Build history of the part. All positions in model axes, mm. A direction names the side the tool comes from. Give positions to 0.01 mm unless a question says otherwise; leave off trailing zeros. Loops run counter-clockwise (first coordinate to the right, second up) from the corner with the lowest first, then second, coordinate; pieces in that order, holes last. Notation, with made-up numbers: (-24.75, 6) -> (34.25, 6) arc R13 ccw to (34.25, 21) -> close; hole circle Ø3 at (44, 37.25). An arc over 180 degrees is marked (long way). Answer as a JSON object with one key per item and string values. Group by question number.
from build123d import *

# Parameters (mm, degrees)
F0_R     = 2.5
F1_DEPTH = 10
F2_DEPTH = 10
F3_R     = 1


with BuildPart() as f1:
    # F0 (on Top) → F1 (new body)
    with BuildSketch(Plane.XY):
        Polygon((-4.778127, 51.351744), (-24.778127, 51.351744), (-24.778127, -18.648256), (40.221873, -18.648256), (40.221873, 51.351744), (20.221873, 51.351744), (20.221873, 1.351744), (-4.778127, 1.351744), align=None)
        with Locations((-14.778127, 18.851744)):
            Circle(F0_R, mode=Mode.SUBTRACT)
        with Locations((30.221873, 18.851744)):
            Circle(F0_R, mode=Mode.SUBTRACT)
    extrude(amount=F1_DEPTH)

    # F0 (on Top) → F2 (join)
    with BuildSketch(Plane.XY):
        Polygon((-4.778127, 51.351744), (-24.778127, 51.351744), (-24.778127, -18.648256), (40.221873, -18.648256), (40.221873, 51.351744), (20.221873, 51.351744), (20.221873, 1.351744), (-4.778127, 1.351744), align=None)
        with Locations((-14.778127, 18.851744)):
            Circle(F0_R, mode=Mode.SUBTRACT)
        with Locations((30.221873, 18.851744)):
            Circle(F0_R, mode=Mode.SUBTRACT)
    extrude(amount=F2_DEPTH)

    # F3
    f3_edges = [f1.edges().sort_by_distance(p)[0] for p in [
        (-14.778127, 51.351744, 10),
        (-24.778127, 16.351744, 10),
        (7.721873, -18.648256, 10),
        (40.221873, 16.351744, 10),
        (30.221873, 51.351744, 10),
        (20.221873, 26.351744, 10),
        (7.721873, 1.351744, 10),
        (-4.778127, 26.351744, 10),
        (-17.278127, 18.851744, 10),
        (27.721873, 18.851744, 10),
    ]]
    fillet(f3_edges, radius=F3_R)


solid = f1.part
(1) Pull direction Y, two halves, no side cores. Call faces 1 (the flat face through (7, -18.648, 4)), 2 (the flat face through (30, 51.352, 4)), 3 (the cylindrical face through (-15.32, 16.41, 4.44)): pulls with the +Y half, pulls with the -Y half, needs draft (parallel to the pull), parting line crosses it, or undercut.
(2) Pin check, flat tips, straight feed: pin 1 (2 mm diameter, centred on x = 16.5, z = 5, fed in from +Y); pin 2 (3 mm diameter, centred on x = -4.5, y = -4.5, fed in from -Z); pin 3 (4 mm diameter, centred on x = -14.78, y = 18.85, fed in from +Z). Stop position of each tip, or through.
(3) Saw through at C-C on z = 3.5. List the corners of the cut face in (x, y).
(4) Saw through at B-B on x = 16.5. List the corners of the cut face in (y, z).
(5) Saw through at A-A on y = 32.5. List the corners of the cut face in (x, z).
(6) 3-axis set-ups, long thin cutter, end or side, ignore diameter. For faces 4 (the flat face through (-24.778, 17, 4)), 5 (the flat face through (20.222, 27, 4)): which of +Z, -Z, +X, -X, +Y, -Y reach the whole face in a straight line?
(7) Probe line 1 along X through (y, z) = (27, 9); line 2 along Y through (x, z) = (-14.5, 4.75); line 3 along X through (y, z) = (21, 2.5). List the from-to ranges inside material, lowest first. Write a range as [from, to].
Calculated:
{
 "1": {"face 1": "pulls with the -Y half", "face 2": "pulls with the +Y half", "face 3": "undercut"},
 "2": {"pin 1": "stops at y = 1.35", "pin 2": "stops at z = 0", "pin 3": "passes through"},
 "3": {"outline": "(-24.78, -18.65) -> (40.22, -18.65) -> (40.22, 51.35) -> (20.22, 51.35) -> (20.22, 1.35) -> (-4.78, 1.35) -> (-4.78, 51.35) -> (-24.78, 51.35) -> close; hole circle Ø5 at (-14.78, 18.85); hole circle Ø5 at (30.22, 18.85)"},
 "4": {"outline": "(-18.65, 0) -> (1.35, 0) -> (1.35, 9) arc R1 ccw to (0.35, 10) -> (-17.65, 10) arc R1 ccw to (-18.65, 9) -> close"},
 "5": {"outline": "(-24.78, 0) -> (-4.78, 0) -> (-4.78, 9) arc R1 ccw to (-5.78, 10) -> (-23.78, 10) arc R1 ccw to (-24.78, 9) -> close; (20.22, 0) -> (40.22, 0) -> (40.22, 9) arc R1 ccw to (39.22, 10) -> (21.22, 10) arc R1 ccw to (20.22, 9) -> close"},
 "6": {"face 4": "+Z, -Z, -X, +Y, -Y", "face 5": "+Z, -Z, +Y"},
 "7": {"line 1": "x = [-24.78, -4.78], [20.22, 40.22]", "line 2": "y = [-18.65, 16.37], [21.34, 51.35]", "line 3": "x = [-24.78, -16.06], [-13.5, -4.78], [20.22, 28.94], [31.5, 40.22]"}
}
